from build123d import *

# Parameters (mm, degrees)
CYLINDER005_R     = 6.5
CYLINDER005_DEPTH = 10
CYLINDER004_R     = 8.2
CYLINDER004_DEPTH = 5
BOX_W             = 10
BOX_H             = 26.4
BOX_DEPTH         = 26.4
FILLET_R          = 10
CYLINDER010_R     = 5.6
CYLINDER010_DEPTH = 10.2
CYLINDER008_R     = 2.2
CYLINDER008_DEPTH = 20
CYLINDER002_R     = 2.2
CYLINDER002_DEPTH = 20
PAD_DEPTH         = 20
PAD001_DEPTH      = 5
CYLINDER009_R     = 5
CYLINDER009_DEPTH = 9.8


with BuildPart() as bring_holder_hole:
    # Cylinder005 → Cylinder005 (new body)
    with BuildSketch(Plane(origin=(0, 0, 0), x_dir=(0, 0, -1), z_dir=(1, 0, 0))):
        Circle(CYLINDER005_R)
    extrude(amount=CYLINDER005_DEPTH)


with BuildPart() as bring_holder_extract:
    # Cylinder004 → Cylinder004 (new body)
    with BuildSketch(Plane(origin=(0, 0, 0), x_dir=(0, 0, -1), z_dir=(1, 0, 0))):
        Circle(CYLINDER004_R)
    extrude(amount=CYLINDER004_DEPTH)

    # Fusion001: union bring holder hole
    add(bring_holder_hole.part)


with BuildPart() as bring_holder_cut:
    # Box → Box (new body)
    with BuildSketch(Plane(origin=(0, -13.2, -13.2), x_dir=(1, 0, 0), z_dir=(0, 0, 1))):
        with Locations((5, 13.2)):
            Rectangle(BOX_W, BOX_H)
    extrude(amount=BOX_DEPTH)

    # Fillet
    fillet_edges = [bring_holder_cut.edges().sort_by_distance(p)[0] for p in [
        (5, -13.2, 13.2),
        (5, 13.2, -13.2),
        (5, 13.2, 13.2),
    ]]
    fillet(fillet_edges, radius=FILLET_R)

    # Cut023015003: cut bring holder extract
    add(bring_holder_extract.part, mode=Mode.SUBTRACT)


with BuildPart() as bring_holder_cut_1:
    # Cut023015003 placement: moved
    add(bring_holder_cut.part.moved(Location((-5, 26, 13.2))))


with BuildPart() as horizontal_body_space:
    # Cylinder010 → Cylinder010 (new body)
    with BuildSketch(Plane(origin=(18, 0, 9.8), x_dir=(1, 0, 0), z_dir=(0, 0, 1))):
        Circle(CYLINDER010_R)
    extrude(amount=CYLINDER010_DEPTH)


with BuildPart() as horizontal_insert_hole:
    # Cylinder008 → Cylinder008 (new body)
    with BuildSketch(Plane(origin=(18, 0, 0), x_dir=(1, 0, 0), z_dir=(0, 0, 1))):
        Circle(CYLINDER008_R)
    extrude(amount=CYLINDER008_DEPTH)


with BuildPart() as f_25_mm_attachment_extract:
    # Cylinder002 → Cylinder002 (new body)
    with BuildSketch(Plane(origin=(-22, 20, 10), x_dir=(1, 0, 0), z_dir=(0, -1, 0))):
        Circle(CYLINDER002_R)
    extrude(amount=CYLINDER002_DEPTH)

    # Fusion007: union horizontal body space, horizontal insert hole
    add(horizontal_body_space.part)
    add(horizontal_insert_hole.part)


with BuildPart() as f_25_mm_attachment_body:
    # Sketch → Pad (new body)
    with BuildSketch(Plane.XY):
        with BuildLine():
            ThreePointArc((12.611106, 1.5), (0, 12.7), (-12.611106, 1.5))
            Line((-22.7, 1.5), (-12.611106, 1.5))
            Line((-22.7, 1.5), (-22.7, 6.5))
            Line((-22.7, 6.5), (-21.463293, 6.5))
            Line((-21.463293, 6.5), (-13.988671, 10.84468))
            ThreePointArc((13.988671, 10.84468), (0, 17.7), (-13.988671, 10.84468))
            Line((13.988671, 10.84468), (21.463293, 6.5))
            Line((21.463293, 6.5), (22.7, 6.5))
            Line((22.7, 6.5), (22.7, 1.5))
            Line((12.611106, 1.5), (22.7, 1.5))
        make_face()
    extrude(amount=PAD_DEPTH)

    # Sketch001 → Pad001 (join)
    with BuildSketch(Plane.XZ.offset(-1.5)):
        with BuildLine():
            Line((-12.611106, 20), (-22.7, 20))
            ThreePointArc((-22.7, 20), (-27.649747, 17.949747), (-29.7, 13))
            Line((-29.7, 13), (-29.7, 7))
            ThreePointArc((-29.7, 7), (-27.649747, 2.050253), (-22.7, 0))
            Line((-12.611106, 0), (-22.7, 0))
            Line((-12.611106, 20), (-12.611106, 0))
        make_face()
    extrude(amount=-PAD001_DEPTH)


with BuildPart() as f_25_mm_16mm_bring_attachment_fusion:
    # Cylinder009 → Cylinder009 (new body)
    with BuildSketch(Plane(origin=(18, 0, 0), x_dir=(1, 0, 0), z_dir=(0, 0, 1))):
        Circle(CYLINDER009_R)
    extrude(amount=CYLINDER009_DEPTH)

    # Fusion006: union 25 mm attachment body
    add(f_25_mm_attachment_body.part)

    # Cut023015002: cut 25 mm attachment extract
    add(f_25_mm_attachment_extract.part, mode=Mode.SUBTRACT)

    # Fusion002: union bring holder cut
    add(bring_holder_cut_1.part)


with BuildPart() as part_mirroring003:
    # Part__Mirroring003: instance of 25 mm 16mm bring attachment fusion
    add(f_25_mm_16mm_bring_attachment_fusion.part.mirror(Plane(origin=(0, 0, 0), x_dir=(0, 1, 0), z_dir=(0, 0, 1))))


solid = part_mirroring003.part
Could you check a few things on this model? Use its own coordinates, in mm. A direction names the side the tool comes from. Coordinates: 2 decimals unless noted, no trailing zeros. Order: outer loops, then holes, each group sorted by start corner. A loop starts at its lowest first (then second) coordinate and runs counter-clockwise, first axis right, second up. Notation, with made-up numbers: (-35, 40.5) -> (13, 40.5) arc R14 ccw to (13, 53.5) -> close; hole circle Ø5 at (87, 80). An arc over 180 degrees is marked (long way). One line per item, written item: value. Start each with the question number.
1) Imagine slicing it at B-B on x = 18. List the corners of the cut face in (y, z) for me.
2) I'm going to push flat-ended pins straight in: pin 1 (1 mm diameter, centred on x = 12.5, z = -10.5, fed in from -Y); pin 2 (6 mm diameter, centred on x = 0, z = -5, fed in from -Y); pin 3 (12 mm diameter, centred on y = 27, z = -18, fed in from -X); pin 4 (3.5 mm diameter, centred on x = -22, z = -10, fed in from +Y). Where does each tip first touch, or does it pass through?
3) Imagine slicing it at A-A on y = 0. List the corners of the cut face in (x, z) for me.
4) Imagine slicing it at C-C on x = 3. List the corners of the cut face in (y, z) for me.
5) If I drill on L1, parallel to Z at x = 1.3, y = 26; L2, parallel to X at y = 0, z = -2.75; L3, parallel to X at y = 5.8, z = -10, over which ranges is the centre line in solid material (lowest first)? Write a range as [from, to].
6) We'd pull the mould along X, two halves only. Please class faces 4 (the flat face through (18, 3, -9.8)), 5 (the flat face through (0, 39.2, -13)), 6 (the flat face through (-17.78, 8.64, -9.86)): +X half, -X half, draft (parallel to the pull), parting line (faces both ways), or undercut.
7) Which directions (+Z, -Z, +X, -X, +Y, -Y) give clear straight access to the entire face, cutting with the end or side of a thin tool? Please do faces 1 (the cylindrical face through (17.25, 5.55, -14.83)), 2 (the flat face through (22.7, 4, -10)), 3 (the flat face through (-29.7, 4, -10)).
8) Imagine slicing it at D-D on y = 31. List the corners of the cut face in (x, z) for me.
Answer list:
1. outline: (-5, -9.8) -> (-2.2, -9.8) -> (-2.2, 0) -> (-5, 0) -> close; (2.2, -9.8) -> (5.6, -9.8) -> (5.6, -20) -> (8.51, -20) -> (8.51, 0) -> (2.2, 0) -> close
2. pin 1: stops at y = 1.52
2. pin 2: stops at y = 12.34
2. pin 3: stops at x = -5
2. pin 4: passes through
3. outline: (13, -9.8) -> (15.8, -9.8) -> (15.8, 0) -> (13, 0) -> close; (20.2, -9.8) -> (23, -9.8) -> (23, 0) -> (20.2, 0) -> close
4. outline: (12.34, -20) -> (13.47, -20) arc R10 ccw to (22.8, -26.4) -> (29.2, -26.4) arc R10 ccw to (39.2, -16.4) -> (39.2, -10) arc R10 ccw to (29.2, 0) -> (12.34, 0) -> close; hole circle Ø13 at (26, -13.2)
5. L1: z = [-26.4, -19.7], [-6.7, 0]
5. L2: x = [13, 15.8], [20.2, 23]
5. L3: x = [-29.7, -24.2], [-19.8, -11.3], [11.3, 22.7]
6. face 4: undercut
6. face 5: draft
6. face 6: -X half
7. face 1: -Z, -Y
7. face 2: +Z, -Z, +X, +Y
7. face 3: +Z, -Z, -X, +Y, -Y
8. outline: (-5, -26.24) -> (5, -26.24) -> (5, -17.35) -> (0, -17.35) -> (0, -19.7) -> (-5, -19.7) -> close; (-5, -6.7) -> (0, -6.7) -> (0, -9.05) -> (5, -9.05) -> (5, -0.16) -> (-5, -0.16) -> close
